Geometry check sheet. Reference: the model listing, model coordinates, mm. Face numbers are marked on the shaded views. Round coordinates to 2 decimals unless told otherwise and drop trailing zeros. Loops run counter-clockwise (first coordinate to the right, second up) from the corner with the lowest first, then second, coordinate; pieces in that order, holes last. Notation, with made-up numbers: M 14.5,22.5 L 72.5,22.5 A15 ccw 72.5,51.5 Z; hole C 39.5,-37 d7. An arc over 180 degrees is marked long. Answer in a Markdown table with one row per item. Add a question column.
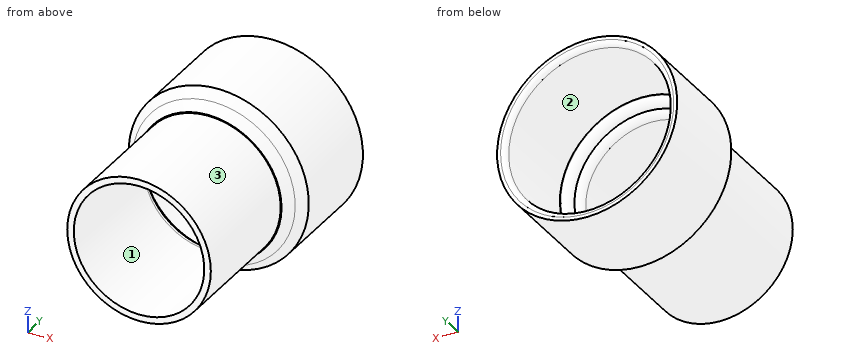
```python
from build123d import *

# Parameters (mm, degrees)
SKETCH1_R                = 41.25
SKETCH1_R_2              = 37.5
BOSS_EXTRUDE2_DEPTH      = 76
SKETCH2_R                = 51.75
SKETCH2_R_2              = 46.75
BOSS_EXTRUDE3_DEPTH      = 60
BOSS_EXTRUDE5_DEPTH      = 5
BOSS_EXTRUDE5_DEPTH_BACK = 5
SKETCH3_R                = 46.75
SKETCH3_R_2              = 41.25
CHAMFER1_SIZE            = 5
CHAMFER2_SIZE            = 5
FILLET1_R                = 5
FILLET2_R                = 5
FILLET3_R                = 3


# Some blends are built 0.0001 mm under size
with BuildPart() as part:
    # Sketch1 → Boss-Extrude2 (new body)
    with BuildSketch(Plane(origin=(0, 0, 0), x_dir=(1, 0, 0), z_dir=(0, 1, 0))):
        with Locations(Location((0, 0, 0), (0, 0, 270))):
            Circle(SKETCH1_R)
        with Locations(Location((0, 0, 0), (0, 0, 270))):
            Circle(SKETCH1_R_2, mode=Mode.SUBTRACT)
    extrude(amount=BOSS_EXTRUDE2_DEPTH)



with BuildPart() as body_2:
    # Sketch2 → Boss-Extrude3 (new body)
    with BuildSketch(Plane(origin=(0, 76, 0), x_dir=(1, 0, 0), z_dir=(0, 1, 0))):
        with Locations(Location((0, 0, 0), (0, 0, 270))):
            Circle(SKETCH2_R)
        with Locations(Location((0, 0, 0), (0, 0, 270))):
            Circle(SKETCH2_R_2, mode=Mode.SUBTRACT)
    extrude(amount=BOSS_EXTRUDE3_DEPTH)


with BuildPart() as part_1:
    add(part.part)

    add(body_2.part)  # Boss-Extrude5 merges body 2
    # Sketch3 → Boss-Extrude5 (add, two sides: drawn at the far end of the back side and taken through both)
    with BuildSketch(Plane(origin=(0, 76, 0), x_dir=(1, 0, 0), z_dir=(0, 1, 0)).offset(-BOSS_EXTRUDE5_DEPTH_BACK)):
        with Locations(Location((0, 0, 0), (0, 0, 270))):
            Circle(SKETCH3_R)
        with Locations(Location((0, 0, 0), (0, 0, 270))):
            Circle(SKETCH3_R_2, mode=Mode.SUBTRACT)
    extrude(amount=BOSS_EXTRUDE5_DEPTH + BOSS_EXTRUDE5_DEPTH_BACK)

    # Chamfer1
    chamfer1_edges = [part_1.edges().sort_by_distance(p)[0] for p in [
        (0, 71, -46.75),
    ]]
    chamfer(chamfer1_edges, length=CHAMFER1_SIZE - 0.0001)  # a hair under: the kernel refuses the full size

    # Chamfer2
    chamfer2_edges = [part_1.edges().sort_by_distance(p)[0] for p in [
        (0, 76, -51.75),
    ]]
    chamfer(chamfer2_edges, length=CHAMFER2_SIZE - 0.0001)  # a hair under: the kernel refuses the full size

    # Fillet1
    fillet1_edges = [part_1.edges().sort_by_distance(p)[0] for p in [
        (0, 81, -41.25),
    ]]
    fillet(fillet1_edges, radius=FILLET1_R - 0.0001)  # a hair under: the kernel refuses the full size

    # Fillet2
    # the kernel refuses this fillet: 5 mm, written as the material it takes off along each edge
    with BuildSketch(Plane(origin=(0, 76, 0), x_dir=(0, 0, 1), z_dir=(-1, 0, 0))) as fillet2_piece_1:
        with BuildLine():
            CenterArc((42.5, -4.841229183), FILLET2_R, 104.477512186, 75.522487814)
            Line((37.5, -4.841229183), (37.4, -4.841229183))
            Line((37.4, -4.841229183), (37.4, 0))
            Line((37.4, 0), (37.5, 0.1))
            ThreePointArc((37.5, 0.1), (39.375, 0.1), (41.225, 0.096824584))
            Line((41.225, 0.096824584), (41.25, 0))
        make_face()
    revolve(axis=Axis((0, 76, 0), (0, 1, 0)), mode=Mode.SUBTRACT)

    # Fillet3
    fillet3_edges = [part_1.edges().sort_by_distance(p)[0] for p in [
        (0, 136, -46.75),
    ]]
    fillet(fillet3_edges, radius=FILLET3_R)


solid = part_1.part
```
1) Thickness scan on L1, parallel to X at y = 40.5, z = 0; L2, parallel to X at y = 116, z = 0; L3, parallel to Z at x = 15, y = 51.5. Record the ranges inside material, lowest first. Write a range as [from, to].
2) Go/stop test with flat-tipped pins: pin 1 (2 mm diameter, centred on x = -23, y = 119.5, fed in from -Z); pin 2 (2 mm diameter, centred on x = 33, z = 17.5, fed in from +Y); pin 3 (1 mm diameter, centred on x = 21, y = 66.5, fed in from -Z). Record where each tip stops, or that it passes through.
3) Cross-section at D-D, the plane y = 108. Record the boundary of the cut face in (x, z), plus the area to 3 significant figures.
4) Cross-section at C-C, the plane y = 46. Record the boundary of the cut face in (x, z).
5) Draft check along Z on the marked faces 1, 2 and 3. Enter one of: +Z half, -Z half, draft (parallel to the pull), parting line (faces both ways), or undercut.
Worked answers:
| question | item | result |
|---|---|---|
| 1 | L1 | x = [-41.25, -37.5], [37.5, 41.25] |
| 1 | L2 | x = [-51.75, -46.75], [46.75, 51.75] |
| 1 | L3 | z = [-38.43, -34.37], [34.37, 38.43] |
| 2 | pin 1 | stops at z = -46.84 |
| 2 | pin 2 | stops at y = 73.95 |
| 2 | pin 3 | stops at z = -35.8 |
| 3 | outline | C 0,0 d103.5; hole C 0,0 d93.5 |
| 3 | area | 1,550 mm2 |
| 4 | outline | C 0,0 d82.5; hole C 0,0 d75 |
| 5 | face 1 | undercut |
| 5 | face 2 | undercut |
| 5 | face 3 | parting line |
